Design review of the part built by this model. Coordinates are the model's own, in mm. A direction names the side the tool comes from. Give positions to 0.01 mm unless a question says otherwise; leave off trailing zeros. Write each loop counter-clockwise with the first axis right and the second up, starting at its lowest first coordinate (ties: lowest second). Pieces come first, ordered by that corner, then holes.
```python
from build123d import *

# Parameters (mm, degrees)
F0_W      = 50.8
F0_H      = 50.8
F1_DEPTH  = 7.62
F2_T      = -2.54
F3_W      = 2.044051
F3_H      = 16.352408
F4_DEPTH  = 6.35
F5_W      = 2.141385
F5_H      = 10.122921
F5_W_2    = 6.813503
F5_H_2    = 1.557372
F6_DEPTH  = 7.62
F7_W      = 1.752042
F7_H      = 7.008177
F8_DEPTH  = 7.62
F9_R      = 1.27
F10_DEPTH = 25.4
F11_R     = 1.27
F12_DEPTH = 25.4


with BuildPart() as f1:
    # F0 (on Top) → F1 (new body)
    with BuildSketch(Plane.XY):
        with Locations((25.4, 25.4)):
            Rectangle(F0_W, F0_H)
    extrude(amount=F1_DEPTH)

    # F2
    f2_openings = [f1.faces().sort_by_distance(p)[0] for p in [
        (25.4, 25.4, 7.62),
    ]]
    offset(amount=F2_T, openings=f2_openings)

    # F3 (on Top) → F4 (join)
    with BuildSketch(Plane.XY):
        Polygon((9.733576, 41.854382), (9.733576, 2.725402), (11.874964, 2.725402), (11.874964, 24.723284), (11.874964, 26.280658), (11.874964, 41.854382), align=None)
        Polygon((11.874964, 26.280658), (11.874964, 24.723284), (21.705878, 24.723284), (23.749929, 24.723284), (31.536791, 24.723284), (31.536791, 26.280658), (28.422045, 26.280658), (26.280656, 26.280658), align=None)
        with Locations((22.727903, 16.54708)):
            Rectangle(F3_W, F3_H)
        Polygon((26.280656, 41.854382), (26.280656, 26.280658), (28.422045, 26.280658), (28.422045, 32.315474), (28.422045, 34.06752), (28.422045, 41.854382), align=None)
        Polygon((28.422045, 34.06752), (28.422045, 32.315474), (32.899488, 32.315474), (35.819563, 32.315474), (43.217082, 32.315474), (43.217082, 34.06752), align=None)
        Polygon((35.819563, 32.315474), (32.899488, 32.315474), (32.899488, 11.874964), (35.819563, 11.874964), (35.819563, 22.095219), (35.819563, 24.723284), align=None)
    extrude(amount=F4_DEPTH)

    # F5 (on Top) → F6 (join)
    with BuildSketch(Plane.XY):
        with Locations((18.007117, 43.411752)):
            Rectangle(F5_W, F5_H)
        with Locations((44.871788, 21.997884)):
            Rectangle(F5_W_2, F5_H_2)
    extrude(amount=F6_DEPTH)

    # F7 (on Top) → F8 (join)
    with BuildSketch(Plane.XY):
        with Locations((38.836971, 44.579783)):
            Rectangle(F7_W, F7_H)
    extrude(amount=F8_DEPTH)

    # F9 (on Top) → F10 (cut)
    with BuildSketch(Plane.XY):
        with Locations((5.645474, 7.008175)):
            Circle(F9_R)
        with Locations((6.034818, 13.042993)):
            Circle(F9_R)
        with Locations((44.19044, 42.633064)):
            Circle(F9_R)
    extrude(amount=F10_DEPTH, mode=Mode.SUBTRACT)

    # F11 (on Top) → F12 (cut)
    with BuildSketch(Plane.XY):
        with Locations((27.254015, 18.299123)):
            Circle(F11_R)
    extrude(amount=F12_DEPTH, mode=Mode.SUBTRACT)


solid = f1.part
```
(1) To check wall thickness, follow L1, parallel to X at y = 42, z = 3.25; L2, parallel to Y at x = 26.5, z = 3.75; L3, parallel to Y at x = 34.5, z = 3. State the ranges of each line that lie inside material, in increasing order.
Resolved:
L1: x = 0 to 2.54, 16.94 to 19.08, 37.96 to 39.71, 48.26 to 50.8
L2: y = 0 to 2.54, 24.72 to 41.85, 48.26 to 50.8
L3: y = 0 to 2.54, 11.87 to 34.07, 48.26 to 50.8
(2) Mouldability with a two-part tool opening along X and no side actions: class faces 3 (the face through (28, 24.723, 4)), 4 (the face through (25, 26, 0)) as pulls with the +X half, pulls with the -X half, needs draft (parallel to the pull), parting line crosses it, or undercut.
Resolved:
face 3: undercut
face 4: needs draft
(3) Clearance check with flat-ended pins moving along their axes: P1, Ø1, axis at x = 44.5, y = 35.5, coming from the -Z side; P2, Ø3, axis at x = 44.19, y = 42.63, coming from the +Z side. State where each tip first meets the part, or that it passes through.
Resolved:
P1: stops at z = 0
P2: stops at z = 2.54
(4) Consider section A-A, the plane z = 3.75. Give the number of separate pieces and of enclosed holes in the cut face, then the cut area to 3 significant figures.
Resolved:
separate pieces: 3
enclosed holes: 1
area: 801 mm2
(5) Consider section D-D, the plane y = 33. Give the boundary of the cut face in (x, z), then the cut area to 3 significant figures.
Resolved:
outline: (0, 0) - (50.8, 0) - (50.8, 7.62) - (48.26, 7.62) - (48.26, 2.54) - (43.22, 2.54) - (43.22, 6.35) - (26.28, 6.35) - (26.28, 2.54) - (11.87, 2.54) - (11.87, 6.35) - (9.73, 6.35) - (9.73, 2.54) - (2.54, 2.54) - (2.54, 7.62) - (0, 7.62) - close
area: 228 mm2
(6) Consider section C-C, the plane x = 3.5. Give the boundary of the cut face in (y, z).
Resolved:
outline: (0, 0) - (50.8, 0) - (50.8, 7.62) - (48.26, 7.62) - (48.26, 2.54) - (2.54, 2.54) - (2.54, 7.62) - (0, 7.62) - close
(7) Consider section B-B, the plane y = 45.5. Give the boundary of the cut face in (x, z), then the cut area to 3 significant figures.
Resolved:
outline: (0, 0) - (50.8, 0) - (50.8, 7.62) - (48.26, 7.62) - (48.26, 2.54) - (39.71, 2.54) - (39.71, 7.62) - (37.96, 7.62) - (37.96, 2.54) - (19.08, 2.54) - (19.08, 7.62) - (16.94, 7.62) - (16.94, 2.54) - (2.54, 2.54) - (2.54, 7.62) - (0, 7.62) - close
area: 175 mm2
(8) Tool access review of faces 1 (the face through (36, 34.068, 4)), 2 (the face through (44.873, 43.704, 1.252)): name each direction out of +Z, -Z, +X, -X, +Y, -Y from which nothing blocks a thin tool from reaching the whole face with its end or side.
Resolved:
face 1: +Z
face 2: +Z, -Z
